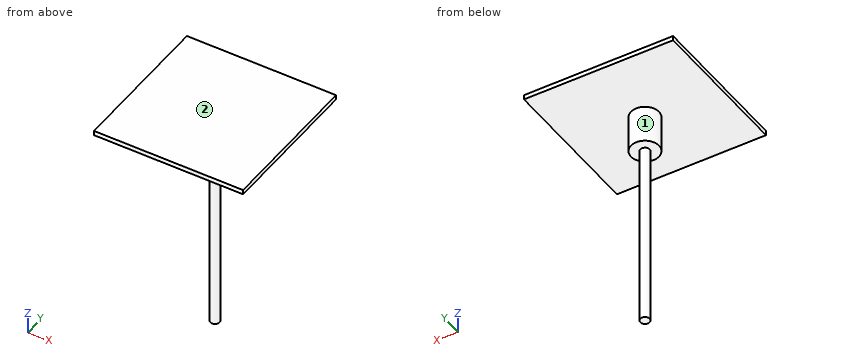
```python
from build123d import *

# Parameters (mm, degrees)
F0_R     = 25
F1_DEPTH = 1000
F2_R     = 75
F2_R_2   = 25
F3_DEPTH = 200
F4_W     = 800
F4_H     = 800
F5_DEPTH = 25


with BuildPart() as f1:
    # F0 (on Top) → F1 (new body)
    with BuildSketch(Plane.XY):
        Circle(F0_R)
    extrude(amount=F1_DEPTH)

    # F2 (on face) → F3 (join)
    with BuildSketch(Plane.XY.offset(1000)):
        Circle(F2_R)
        Circle(F2_R_2, mode=Mode.SUBTRACT)
        Circle(F2_R_2)
    extrude(amount=F3_DEPTH)

    # F4 (on face) → F5 (join)
    with BuildSketch(Plane.XY.offset(1200)):
        Rectangle(F4_W, F4_H)
    extrude(amount=F5_DEPTH)


solid = f1.part
```
Design review of the part built by this model. Coordinates are the model's own, in mm. Face numbers are marked on the shaded views. A direction names the side the tool comes from. Round coordinates to 2 decimals unless told otherwise and drop trailing zeros. Write each loop counter-clockwise with the first axis right and the second up, starting at its lowest first coordinate (ties: lowest second). Pieces come first, ordered by that corner, then holes.
Item 1: We need section C-C on y = -298. Write out the cut boundary in (x, z).
Item 2: For probe 1 along Z at (x, y) = (-64, -43.5); probe 2 along Y at (x, z) = (-43.5, 1050.5); probe 3 along X at (y, z) = (-6.5, 501), list the stretches that pass through material, from the lowest coordinate up.
Item 3: For the marked faces 1 and 2, list the 3-axis set-ups (+Z, -Z, +X, -X, +Y, -Y) from which the entire face can be reached by the end or side of a thin tool; tool diameter is ignored.
Item 4: Clearance check with flat-ended pins moving along their axes: pin 1 Ø1 at (x, y) = (-251, -254.5) entering from -Z; pin 2 Ø3 at (y, z) = (-31, 1003.5) entering from -X. State where each tip first meets the part, or that it passes through.
Item 5: We need section A-A on x = 0. Write out the cut boundary in (y, z).
Returned:
1. outline: (-400, 1200) - (400, 1200) - (400, 1225) - (-400, 1225) - close
2. probe 1: z = 1200 to 1225
2. probe 2: y = -61.1 to 61.1
2. probe 3: x = -24.14 to 24.14
3. face 1: -Z
3. face 2: +Z, +X, -X, +Y, -Y
4. pin 1: stops at z = 1200
4. pin 2: stops at x = -68.95
5. outline: (-400, 1200) - (-75, 1200) - (-75, 1000) - (-25, 1000) - (-25, 0) - (25, 0) - (25, 1000) - (75, 1000) - (75, 1200) - (400, 1200) - (400, 1225) - (-400, 1225) - close
